Can you work these out from the model? Positions are in its coordinate system, mm. A direction names the side the tool comes from. Give positions to 0.01 mm unless a question says otherwise; leave off trailing zeros. Order: outer loops, then holes, each group sorted by start corner. A loop starts at its lowest first (then second) coordinate and runs counter-clockwise, first axis right, second up.
```python
from build123d import *

# Parameters (mm, degrees)
SKETCH001_W  = 0.5
SKETCH001_H  = 5.5
PAD001_DEPTH = 0.19
PAD_DEPTH    = 8


with BuildPart() as pad001:
    # Sketch001 → Pad001 (new body, symmetric)
    with BuildSketch(Plane.XZ):
        with Locations((2.54, 0.05)):
            Rectangle(SKETCH001_W, SKETCH001_H)
        Polygon((0.25, -2.7), (-0.25, -2.7), (-0.25, 0.26), (1.02, 2.16), (1.02, 2.8), (1.52, 2.8), (1.52, 2.16), (0.25, 0.26), align=None)
        Polygon((3.56, 2.8), (4.06, 2.8), (4.06, 2.16), (5.33, 0.26), (5.33, -2.7), (4.83, -2.7), (4.83, 0.26), (3.56, 2.16), align=None)
    extrude(amount=PAD001_DEPTH, both=True)


with BuildPart() as to_92l_inline_wide:
    # Sketch → Pad (new body)
    with BuildSketch(Plane.XY.offset(2.5)):
        with BuildLine():
            Line((0.524231, -1.33), (4.555769, -1.33))
            ThreePointArc((4.555769, -1.33), (2.54, 2.415), (0.524231, -1.33))
        make_face()
    extrude(amount=PAD_DEPTH)

    add(pad001.part)


solid = to_92l_inline_wide.part
```
1) Suppose I cut it at B-B (y = 0). Please give me the cut outline in (x, z) (3 decimals), and give its area (3 significant figures).
2) Suppose I cut it at C-C (x = 0.65). Please give me the cut outline in (y, z), and give its area (3 significant figures).
3) Suppose I cut it at A-A (x = 2.54). Please give me the cut outline in (y, z) (3 decimals), and give its area (3 significant figures).
4) If I drill on line 1 (X direction, y = 0.15, z = -1.5); line 2 (Z direction, x = 2.15, y = -0.15); line 3 (Y direction, x = 4.9, z = 0.25), over which ranges is the centre line in solid material (lowest first)?
5) I'm going to push flat-ended pins straight in: pin 1 Ø2 at (y, z) = (1, 4.5) entering from +X (3 decimals); pin 2 Ø0.9 at (x, z) = (0.5, -0.5) entering from -Y; pin 3 Ø1.4 at (x, z) = (5, 1) entering from +Y. Where does each tip first touch, or does it pass through?
6) Which directions (+Z, -Z, +X, -X, +Y, -Y) give clear straight access to the entire face, cutting with the end or side of a thin tool? Please do faces 5 (the face through (3, -1.33, 6)), 6 (the face through (0, -0.19, 0)), 7 (the face through (4.2, 0, 1.2)), 8 (the face through (5, 0.19, 0)), 9 (the face through (0.38, 0, 1.2)).
7) We'd pull the mould along Z, two halves only. Please class faces 1 (the face through (3, 1, 10.5)), 2 (the face through (4.7, 0, 1.2)), 3 (the face through (2.613, 2.414, 6.444)), 4 (the face through (0.89, 0, 1.22)): +Z half, -Z half, draft (parallel to the pull), parting line (faces both ways), or undercut.
8) Suppose I cut it at D-D (z = 0.5). Please give me the cut outline in (x, y).
Results:
1. outline: (-0.25, -2.7) - (0.25, -2.7) - (0.25, 0.26) - (1.52, 2.16) - (1.52, 2.5) - (2.29, 2.5) - (2.29, -2.7) - (2.79, -2.7) - (2.79, 2.5) - (3.56, 2.5) - (3.56, 2.16) - (4.83, 0.26) - (4.83, -2.7) - (5.33, -2.7) - (5.33, 0.26) - (4.06, 2.16) - (4.06, 2.5) - (4.955, 2.5) - (4.955, 10.5) - (0.125, 10.5) - (0.125, 2.5) - (1.02, 2.5) - (1.02, 2.16) - (-0.25, 0.26) - close
1. area: 46.4 mm2
2. outline: (-1.33, 2.5) - (1.5, 2.5) - (1.5, 10.5) - (-1.33, 10.5) - close; (-0.19, 0.86) - (0.19, 0.86) - (0.19, 1.61) - (-0.19, 1.61) - close
2. area: 23.0 mm2
3. outline: (-1.33, 2.5) - (-0.19, 2.5) - (-0.19, -2.7) - (0.19, -2.7) - (0.19, 2.5) - (2.415, 2.5) - (2.415, 10.5) - (-1.33, 10.5) - close
3. area: 31.9 mm2
4. line 1: x = -0.25 to 0.25, 2.29 to 2.79, 4.83 to 5.33
4. line 2: z = 2.5 to 10.5
4. line 3: y = -0.19 to 0.19
5. pin 1: stops at x = 4.955
5. pin 2: stops at y = -0.19
5. pin 3: stops at y = 0.19
6. face 5: +Z, -Z, +X, -X, -Y
6. face 6: -Z, +X, -X, -Y
6. face 7: -Z, +Y, -Y
6. face 8: -Z, +X, -X, +Y
6. face 9: -X, +Y, -Y
7. face 1: +Z half
7. face 2: undercut
7. face 3: draft
7. face 4: -Z half
8. outline: (-0.09, -0.19) - (0.41, -0.19) - (0.41, 0.19) - (-0.09, 0.19) - close; (2.29, -0.19) - (2.79, -0.19) - (2.79, 0.19) - (2.29, 0.19) - close; (4.67, -0.19) - (5.17, -0.19) - (5.17, 0.19) - (4.67, 0.19) - close
